Part model, mm, in its own coordinate system. A direction names the side the tool comes from. Round coordinates to 2 decimals unless told otherwise and drop trailing zeros. Order: outer loops, then holes, each group sorted by start corner. A loop starts at its lowest first (then second) coordinate and runs counter-clockwise, first axis right, second up. Notation, with made-up numbers: (1.25, 76) -> (51.25, 76) arc R8 ccw to (51.25, 83) -> close; hole circle Ø11 at (45, -9). An arc over 180 degrees is marked (long way). Return JSON: item names as keys, results as strings. Group by question number.
from build123d import *

# Parameters (mm, degrees)
SKETCH1_W           = 127
SKETCH1_H           = 127
BOSS_EXTRUDE1_DEPTH = 15.24
SKETCH2_W           = 127
SKETCH2_H           = 127
SKETCH2_W_2         = 100.33
SKETCH2_H_2         = 100.33
CUT_EXTRUDE1_DEPTH  = 6.35
FILLET1_R           = 0.762
CHAMFER1_SIZE       = 0.762


with BuildPart() as part:
    # Sketch1 → Boss-Extrude1 (new body)
    with BuildSketch(Plane(origin=(0, 0, 0), x_dir=(1, 0, 0), z_dir=(0, 1, 0))):
        Rectangle(SKETCH1_W, SKETCH1_H)
    extrude(amount=BOSS_EXTRUDE1_DEPTH)

    # Sketch2 → Cut-Extrude1 (cut)
    with BuildSketch(Plane.XZ):
        Rectangle(SKETCH2_W, SKETCH2_H)
        Rectangle(SKETCH2_W_2, SKETCH2_H_2, mode=Mode.SUBTRACT)
    extrude(amount=-CUT_EXTRUDE1_DEPTH, mode=Mode.SUBTRACT)

    # Fillet1
    fillet1_edges = [part.edges().sort_by_distance(p)[0] for p in [
        (-50.165, 3.175, -50.165),
        (-50.165, 3.175, 50.165),
        (50.165, 3.175, 50.165),
        (50.165, 3.175, -50.165),
    ]]
    fillet(fillet1_edges, radius=FILLET1_R)

    # Chamfer1
    chamfer1_edges = [part.edges().sort_by_distance(p)[0] for p in [
        (-63.5, 15.24, 0),
        (0, 15.24, 63.5),
        (63.5, 15.24, 0),
        (0, 15.24, -63.5),
    ]]
    chamfer(chamfer1_edges, length=CHAMFER1_SIZE)


solid = part.part
(1) Probe L1, parallel to X at y = 1, z = -29 (3 decimals); L2, parallel to X at y = 14.5, z = -34. List the from-to ranges inside material, lowest first. Write a range as [from, to].
(2) Tool access for faces 1 (the flat face through (-57, 6.35, 1)), 2 (the flat face through (-1, 3, -50.165)), 3 (the flat face through (-1, 3, 50.165)), 4 (the flat face through (50.165, 3, -1)), 5 (the flat face through (-50.165, 3, -1)): list every direction of +Z, -Z, +X, -X, +Y, -Y with a clear straight run to the whole face (end or side of a thin tool).
(3) Pin check, flat tips, straight feed: P1, Ø5, axis at x = 10.5, y = 4, coming from the -Z side; P2, Ø1.9, axis at y = 2.5, z = -14.5, coming from the +X side (3 decimals); P3, Ø3, axis at x = 23.5, y = 4, coming from the +Z side (3 decimals). Stop position of each tip, or through.
(4) Saw through at C-C, the plane z = 14.5. List the corners of the cut face in (x, y) (3 decimals).
(5) Saw through at A-A, the plane y = 1.75. List the corners of the cut face in (x, z) (3 decimals), and give its area (3 significant figures).
(6) Saw through at B-B, the plane x = 15. List the corners of the cut face in (y, z) (3 decimals), and give its area (3 significant figures).
(7) Saw through at D-D, the plane z = -54. List the corners of the cut face in (x, y), and give its area (3 significant figures).
Results are:
{
 "1": {"L1": "x = [-50.165, 50.165]", "L2": "x = [-63.48, 63.48]"},
 "2": {"face 1": "-Y", "face 2": "-Z, +X, -X, -Y", "face 3": "+Z, +X, -X, -Y", "face 4": "+Z, -Z, +X, -Y", "face 5": "+Z, -Z, -X, -Y"},
 "3": {"P1": "stops at z = -63.5", "P2": "stops at x = 50.165", "P3": "stops at z = 50.165"},
 "4": {"outline": "(-63.5, 6.35) -> (-50.165, 6.35) -> (-50.165, 0) -> (50.165, 0) -> (50.165, 6.35) -> (63.5, 6.35) -> (63.5, 14.478) -> (62.738, 15.24) -> (-62.738, 15.24) -> (-63.5, 14.478) -> close"},
 "5": {"outline": "(-50.165, -49.403) arc R0.762 ccw to (-49.403, -50.165) -> (49.403, -50.165) arc R0.762 ccw to (50.165, -49.403) -> (50.165, 49.403) arc R0.762 ccw to (49.403, 50.165) -> (-49.403, 50.165) arc R0.762 ccw to (-50.165, 49.403) -> close", "area": "10,100 mm^2"},
 "6": {"outline": "(0, -50.165) -> (6.35, -50.165) -> (6.35, -63.5) -> (14.478, -63.5) -> (15.24, -62.738) -> (15.24, 62.738) -> (14.478, 63.5) -> (6.35, 63.5) -> (6.35, 50.165) -> (0, 50.165) -> close", "area": "1,770 mm^2"},
 "7": {"outline": "(-63.5, 6.35) -> (63.5, 6.35) -> (63.5, 14.48) -> (62.74, 15.24) -> (-62.74, 15.24) -> (-63.5, 14.48) -> close", "area": "1,130 mm^2"}
}
